```python
from build123d import *

# Parameters (mm, degrees)
SKETCH1_W           = 90
SKETCH1_H           = 90
BOSS_EXTRUDE1_DEPTH = 30
SKETCH2_R           = 4
CUT_EXTRUDE1_DEPTH  = 40
SKETCH3_R           = 12.5
CUT_EXTRUDE2_DEPTH  = 35
SKETCH5_R           = 1.5
CUT_EXTRUDE3_DEPTH  = 40
SKETCH9_R           = 1.5
CUT_EXTRUDE4_DEPTH  = 15


with BuildPart() as part:
    # Sketch1 → Boss-Extrude1 (new body)
    with BuildSketch(Plane.XY):
        Rectangle(SKETCH1_W, SKETCH1_H)
    extrude(amount=BOSS_EXTRUDE1_DEPTH)

    # Sketch2 → Cut-Extrude1 (cut)
    with BuildSketch(Plane.XZ.offset(45)):
        with Locations(Location((-30, 15, 0), (0, 0, 270))):
            Circle(SKETCH2_R)
        with Locations(Location((30, 15, 0), (0, 0, 270))):
            Circle(SKETCH2_R)
    extrude(amount=-CUT_EXTRUDE1_DEPTH, mode=Mode.SUBTRACT)

    # Sketch3 → Cut-Extrude2 (cut)
    with BuildSketch(Plane.XY.offset(30)):
        with BuildLine():
            Line((12.5, -45), (12.5, 0))
            ThreePointArc((12.5, 0), (0, -12.5), (-12.5, 0))
            Line((-12.5, 0), (-12.5, -45))
            Line((-12.5, -45), (12.5, -45))
        make_face()
        Circle(SKETCH3_R)
    extrude(amount=-CUT_EXTRUDE2_DEPTH, mode=Mode.SUBTRACT)

    # Sketch5 → Cut-Extrude3 (cut)
    with BuildSketch(Plane.XY.offset(30)):
        with Locations((-30, 30)):
            Circle(SKETCH5_R)
        with Locations((-33, 15)):
            Circle(SKETCH5_R)
        with Locations((30, 30)):
            Circle(SKETCH5_R)
        with Locations((33, 15)):
            Circle(SKETCH5_R)
        with Locations((39, -33)):
            Circle(SKETCH5_R)
        with Locations((22.5, -33)):
            Circle(SKETCH5_R)
        with Locations((-22.5, -33)):
            Circle(SKETCH5_R)
        with Locations((-39, -33)):
            Circle(SKETCH5_R)
    extrude(amount=-CUT_EXTRUDE3_DEPTH, mode=Mode.SUBTRACT)

    # Sketch9 → Cut-Extrude4 (cut)
    with BuildSketch(Plane.XY.offset(30)):
        with Locations((-30, -20)):
            Circle(SKETCH9_R)
        with Locations((30, -20)):
            Circle(SKETCH9_R)
    extrude(amount=-CUT_EXTRUDE4_DEPTH, mode=Mode.SUBTRACT)


solid = part.part
```
For this review, take the finished solid that the model builds, in its own axes (mm). A direction names the side the tool comes from. Round coordinates to 2 decimals unless told otherwise and drop trailing zeros. Order: outer loops, then holes, each group sorted by start corner. A loop starts at its lowest first (then second) coordinate and runs counter-clockwise, first axis right, second up.
Q1. Machinability: for faces 1 (the flat face through (-12.5, -22, 15)), 2 (the cylindrical face through (-28.799, -25.28, 11.185)), 3 (the cylindrical face through (-31.11, -18.99, 24.43)), which of the approach directions +Z, -Z, +X, -X, +Y, -Y give a long, thin tool a straight path to every point of the face, cutting with its end or side? Answer none if there is none.
Findings below:
face 1: +Z, -Z, -Y
face 2: -Y
face 3: +Z
Q2. Insertion check: P1, Ø4, axis at x = -30, y = -20, coming from the -Z side; P2, Ø1.8, axis at x = -33, y = 15, coming from the +Z side; P3, Ø6, axis at x = 6, z = 14.5, coming from the -Y side. Each pin has a flat end and moves straight along its axis. Give the tip position at first contact, or say it passes through.
Findings below:
P1: stops at z = 0
P2: passes through
P3: stops at y = 8.67
Q3. We need section C-C, the plane x = 22.5. Give the boundary of the cut face in (y, z), plus the area to 3 significant figures.
Findings below:
outline: (-45, 0) - (-34.5, 0) - (-34.5, 30) - (-45, 30) - close; (-31.5, 0) - (45, 0) - (45, 30) - (-31.5, 30) - close
area: 2,610 mm2
Q4. We need section A-A, the plane y = -33. Give the boundary of the cut face in (x, z), plus the area to 3 significant figures.
Findings below:
outline: (-45, 0) - (-40.5, 0) - (-40.5, 30) - (-45, 30) - close; (-37.5, 0) - (-24, 0) - (-24, 30) - (-37.5, 30) - close; (-21, 0) - (-12.5, 0) - (-12.5, 30) - (-21, 30) - close; (12.5, 0) - (21, 0) - (21, 30) - (12.5, 30) - close; (24, 0) - (37.5, 0) - (37.5, 30) - (24, 30) - close; (40.5, 0) - (45, 0) - (45, 30) - (40.5, 30) - close; hole circle Ø8 at (-30, 15); hole circle Ø8 at (30, 15)
area: 1,490 mm2
Q5. Wall thickness on line 1 (X direction, y = -20, z = 22); line 2 (Y direction, x = 39, z = 17); line 3 (X direction, y = -7, z = 12): over which ranges is each line inside the solid? List them lowest first.
Findings below:
line 1: x = -45 to -31.5, -28.5 to -12.5, 12.5 to 28.5, 31.5 to 45
line 2: y = -45 to -34.5, -31.5 to 45
line 3: x = -45 to -32.65, -27.35 to -12.5, 12.5 to 27.35, 32.65 to 45
Q6. Mouldability with a two-part tool opening along Z and no side actions: class faces 4 (the flat face through (30, -5, 15)), 5 (the flat face through (9, 11, 0)), 6 (the cylindrical face through (21.3, -33.9, 15.2)) as pulls with the +Z half, pulls with the -Z half, needs draft (parallel to the pull), parting line crosses it, or undercut.
Findings below:
face 4: undercut
face 5: pulls with the -Z half
face 6: needs draft
Q7. We need section B-B, the plane y = -7. Give the boundary of the cut face in (x, z).
Findings below:
outline: (-45, 0) - (-12.5, 0) - (-12.5, 30) - (-45, 30) - close; (12.5, 0) - (45, 0) - (45, 30) - (12.5, 30) - close; hole circle Ø8 at (-30, 15); hole circle Ø8 at (30, 15)
Q8. We need section D-D, the plane z = 25.5. State how many separate pieces and enclosed holes the cut face has, plus the area to 3 significant figures.
Findings below:
separate pieces: 1
enclosed holes: 10
area: 6,660 mm2
